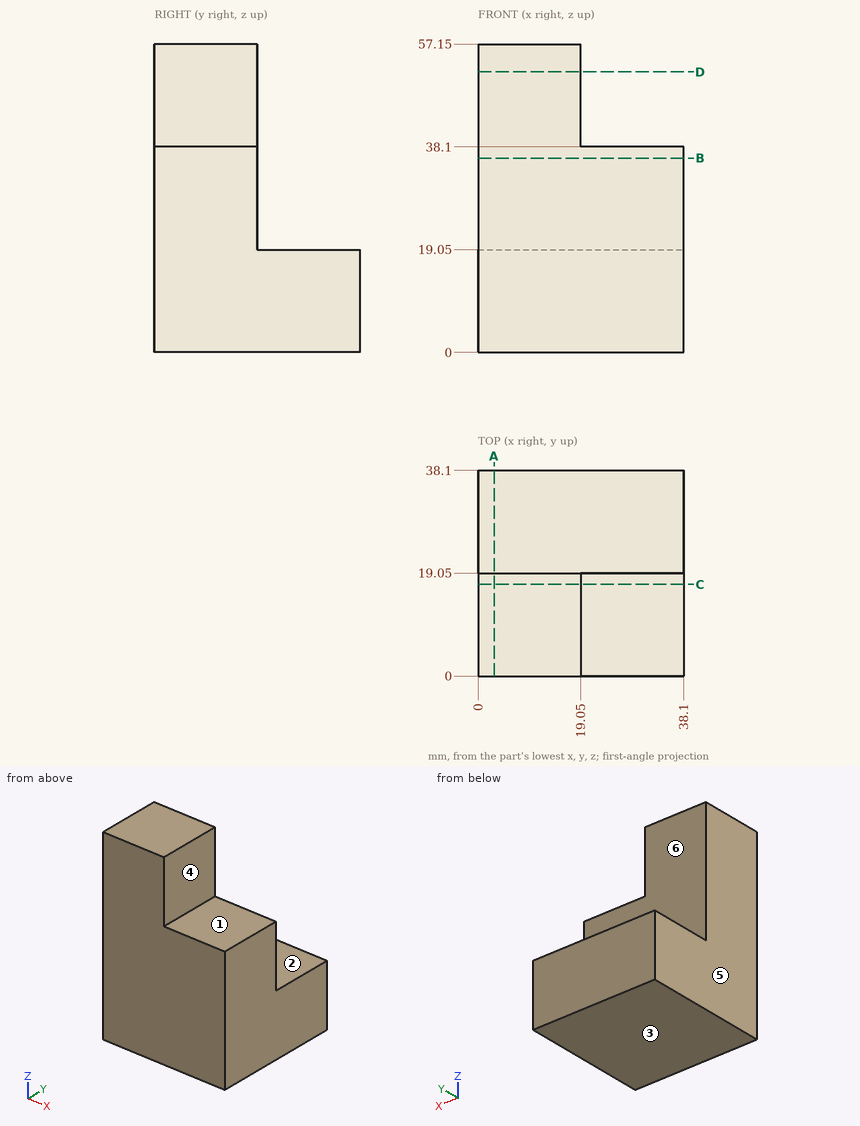
Part print with two shaded views. Sizes in mm from the minimum x, y, z corner. A direction names the side the tool comes from. Coordinates: 2 decimals unless noted, no trailing zeros. Write each loop counter-clockwise with the first axis right and the second up, starting at its lowest first coordinate (ties: lowest second). Pieces come first, ordered by that corner, then holes. Notation, with made-up numbers: (20, 42.5) - (46, 42.5) arc R17 cw to (46, 73.5) - close; hole circle Ø8 at (16, -20.75). An arc over 180 degrees is marked (long way). Use a Markdown table: item, result. Add a question column.
Item 1: Band-saw the part on D-D, the plane z = 52. Write the cut outline in (x, y), and give its area (3 significant figures).
Item 2: 3-axis set-ups, long thin cutter, end or side, ignore diameter. For the marked faces 1, 2 and 3: which of +Z, -Z, +X, -X, +Y, -Y reach the whole face in a straight line?
Item 3: Drop flat-ended pins along their axis: pin 1 (5.5 mm diameter, centred on x = 15.5, y = 29, fed in from +Z); pin 2 (5.5 mm diameter, centred on x = 25.5, y = 9, fed in from +Z); pin 3 (8 mm diameter, centred on x = 13.5, z = 32, fed in from +Y); pin 4 (11.5 mm diameter, centred on x = 25.5, z = 45.5, fed in from +Y). Give the stop position or say it passes through.
Item 4: Drill centre lines: line 1 along Z through (x, y) = (22.5, 9.5); line 2 along Y through (x, z) = (21.5, 20). Where is each one in solid material? Low to high.
Item 5: Two-plate mould, pull along X, no slides. Class the marked faces 4, 5 and 6: pulls with the +X half, pulls with the -X half, needs draft (parallel to the pull), parting line crosses it, or undercut.
Item 6: Band-saw the part on C-C, the plane y = 17. Write the cut outline in (x, z).
Item 7: Band-saw the part on A-A, the plane x = 3. Write the cut outline in (y, z), and give its area (3 significant figures).
Item 8: Band-saw the part on B-B, the plane z = 36. Write the cut outline in (x, y).
A:
| question | item | result |
|---|---|---|
| 1 | outline | (0, 0) - (19.05, 0) - (19.05, 19.05) - (0, 19.05) - close |
| 1 | area | 363 mm² |
| 2 | face 1 | +Z, +X, +Y, -Y |
| 2 | face 2 | +Z, +X, -X, +Y |
| 2 | face 3 | -Z, +X, -X, +Y, -Y |
| 3 | pin 1 | stops at z = 19.05 |
| 3 | pin 2 | stops at z = 38.1 |
| 3 | pin 3 | stops at y = 19.05 |
| 3 | pin 4 | passes through |
| 4 | line 1 | z = 0 to 38.1 |
| 4 | line 2 | y = 0 to 19.05 |
| 5 | face 4 | pulls with the +X half |
| 5 | face 5 | pulls with the -X half |
| 5 | face 6 | needs draft |
| 6 | outline | (0, 0) - (38.1, 0) - (38.1, 38.1) - (19.05, 38.1) - (19.05, 57.15) - (0, 57.15) - close |
| 7 | outline | (0, 0) - (38.1, 0) - (38.1, 19.05) - (19.05, 19.05) - (19.05, 57.15) - (0, 57.15) - close |
| 7 | area | 1,450 mm² |
| 8 | outline | (0, 0) - (38.1, 0) - (38.1, 19.05) - (0, 19.05) - close |
